Source: three-view drawing plus pictorial views. Frame: mm from the lowest corner of the part. A direction names the side the tool comes from. Round coordinates to 2 decimals unless told otherwise and drop trailing zeros. Write each loop counter-clockwise with the first axis right and the second up, starting at its lowest first coordinate (ties: lowest second). Pieces come first, ordered by that corner, then holes. Notation, with made-up numbers: (70.25, 65.25) - (117.25, 65.25) arc R19 ccw to (117.25, 69.25) - close; hole circle Ø8 at (-32.5, 70). An arc over 180 degrees is marked (long way). Write each question's results on one line, items separated by ' | '.
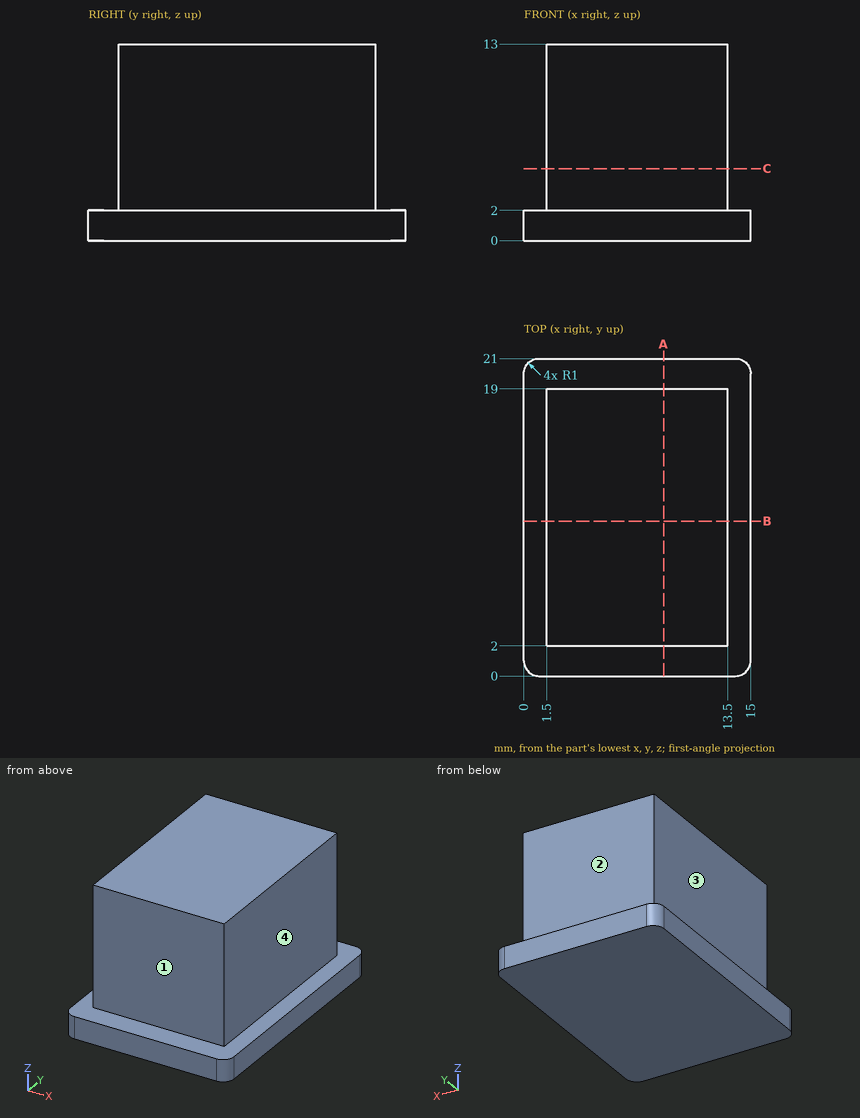
Q1. Section query C-C, the plane z = 4.75. Return loops of the section in (x, y), plus the area to 3 significant figures.
Answer block:
outline: (1.5, 2) - (13.5, 2) - (13.5, 19) - (1.5, 19) - close | area: 204 mm2
Q2. Access query for the marked faces 1, 2, 3 and 4. Directions: +Z, -Z, +X, -X, +Y, -Y. A direction counts if a zero-diameter tool reaches every point of the face in a straight line with its end or side. Return the directions, or none.
Answer block:
face 1: +Z, +X, -X, -Y | face 2: +Z, +X, -X, +Y | face 3: +Z, -X, +Y, -Y | face 4: +Z, +X, +Y, -Y
Q3. Pin query (flat end, axial travel): pin 1 (8 mm diameter, centred on x = 8, y = 15, fed in from -Z); pin 2 (2 mm diameter, centred on y = 4, z = 4, fed in from +X). Return the tip coordinate at first contact, or that it passes through.
Answer block:
pin 1: z = 0 | pin 2: x = 13.5
Q4. Section query A-A, the plane x = 9.25. Return loops of the section in (y, z).
Answer block:
outline: (0, 0) - (21, 0) - (21, 2) - (19, 2) - (19, 13) - (2, 13) - (2, 2) - (0, 2) - close
Q5. Section query B-B, the plane y = 10.25. Return loops of the section in (x, z).
Answer block:
outline: (0, 0) - (15, 0) - (15, 2) - (13.5, 2) - (13.5, 13) - (1.5, 13) - (1.5, 2) - (0, 2) - close
Q6. Ray query, line 1 along Y through (x, z) = (7.5, 5); line 2 along X through (y, z) = (8.75, 8.5); line 3 along Z through (x, y) = (13.25, 20). Return the intervals inside material, ascending.
Answer block:
line 1: 2 to 19 | line 2: 1.5 to 13.5 | line 3: 0 to 2
